Check sheet for the drawn part. Datum: minimum x, y, z corner. Units: mm. A direction names the side the tool comes from. Give positions to 0.01 mm unless a question says otherwise; leave off trailing zeros. Loops run counter-clockwise (first coordinate to the right, second up) from the corner with the lowest first, then second, coordinate; pieces in that order, holes last.
1. Release check for a two-part mould opening along X. For the marked faces 3, 4 and 5 record: +X half, -X half, draft (parallel to the pull), parting line (faces both ways), or undercut.
2. Cross-section at A-A, the plane x = 25. Record the cut outline in (y, z), plus the area to 3 significant figures.
3. Cross-section at B-B, the plane z = 10. Record the cut outline in (x, y) (1 decimal), plus the area to 3 significant figures.
4. Cross-section at C-C, the plane z = 16.25. Record the cut outline in (x, y) (1 decimal), plus the area to 3 significant figures.
5. Material ranges on L1, parallel to Z at x = 25, y = 2; L2, parallel to Y at x = 26, z = 5; L3, parallel to Y at x = 11, z = 16.75 (1 decimal), recorded low to high.
6. Go/stop test with flat-tipped pins: pin 1 Ø2 at (y, z) = (19.5, 18) entering from -X; pin 2 Ø10 at (y, z) = (12, 15) entering from -X; pin 3 Ø8 at (y, z) = (9.5, 3) entering from +X; pin 4 Ø10 at (x, z) = (44.5, 16) entering from -Y. Record where each tip stops, or that it passes through.
7. Cross-section at D-D, the plane x = 45.5. Record the cut outline in (y, z), plus the area to 3 significant figures.
8. Tool access check on the marked faces 1 and 2. Record the directions out of +Z, -Z, +X, -X, +Y, -Y that give a thin tool (end or side, any length) a straight path to the whole face; none if there is none.
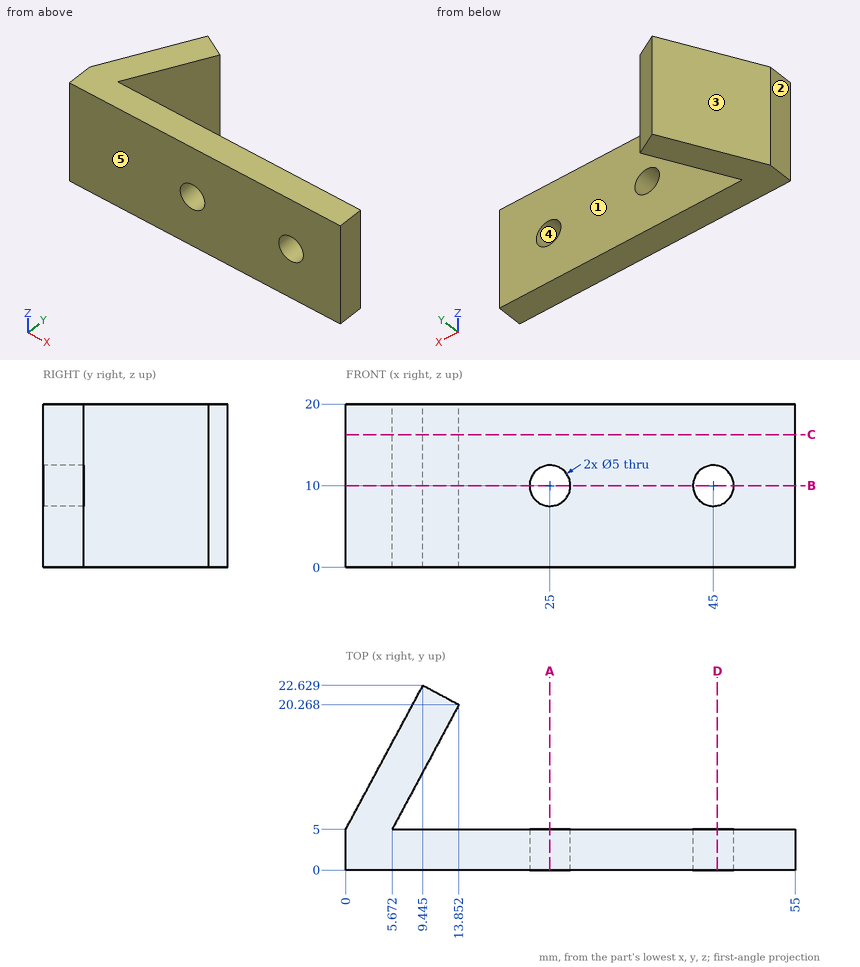
Result:
1. face 3: -X half
1. face 4: undercut
1. face 5: draft
2. outline: (0, 0) - (5, 0) - (5, 7.5) - (0, 7.5) - close; (0, 12.5) - (5, 12.5) - (5, 20) - (0, 20) - close
2. area: 75.0 mm2
3. outline: (0, 0) - (22.5, 0) - (22.5, 5) - (5.7, 5) - (13.9, 20.3) - (9.4, 22.6) - (0, 5) - close; (27.5, 0) - (42.5, 0) - (42.5, 5) - (27.5, 5) - close; (47.5, 0) - (55, 0) - (55, 5) - (47.5, 5) - close
3. area: 318 mm2
4. outline: (0, 0) - (55, 0) - (55, 5) - (5.7, 5) - (13.9, 20.3) - (9.4, 22.6) - (0, 5) - close
4. area: 368 mm2
5. L1: z = 0 to 7.5, 12.5 to 20
5. L2: y = 0 to 5
5. L3: y = 0 to 5, 14.9 to 21.8
6. pin 1: stops at x = 7.23
6. pin 2: stops at x = 1.07
6. pin 3: stops at x = 10.23
6. pin 4: stops at y = 0
7. outline: (0, 0) - (5, 0) - (5, 7.55) - (0, 7.55) - close; (0, 12.45) - (5, 12.45) - (5, 20) - (0, 20) - close
7. area: 75.5 mm2
8. face 1: +Z, -Z, +X
8. face 2: +Z, -Z, -X, +Y, -Y
